from build123d import *

# Parameters (mm, degrees)
SKETCH1_R          = 6.35
BASE_EXTRUDE_DEPTH = 1.5875
CHAMFER1_SIZE      = 0.254


with BuildPart() as part:
    # Sketch1 → Base-Extrude (new body, symmetric)
    with BuildSketch(Plane(origin=(0, 0, 0), x_dir=(1, 0, 0), z_dir=(0, 1, 0))):
        with BuildLine():
            Line((6.35, 0), (6.35, 104.775))
            ThreePointArc((6.35, 104.775), (12.7, 111.125), (19.05, 104.775))
            Line((19.05, 104.775), (19.05, -31.75))
            ThreePointArc((19.05, -31.75), (0, -50.8), (-19.05, -31.75))
            Line((-19.05, -31.75), (-19.05, 104.775))
            ThreePointArc((-19.05, 104.775), (-12.7, 111.125), (-6.35, 104.775))
            Line((-6.35, 104.775), (-6.35, 0))
            ThreePointArc((-6.35, 0), (0, -6.35), (6.35, 0))
        make_face()
        with Locations(Location((0, -31.75, 0), (0, 0, 270))):  # turned: the seam where the file's is
            Circle(SKETCH1_R, mode=Mode.SUBTRACT)
    extrude(amount=BASE_EXTRUDE_DEPTH, both=True)

    # Chamfer1
    chamfer1_edges = [part.edges().sort_by_distance(p)[0] for p in [
        (-12.7, 1.5875, -111.125),
        (-6.35, -1.5875, -52.3875),
        (0, -1.5875, 6.35),
        (-19.05, 1.5875, -36.5125),
        (0, 1.5875, 50.8),
        (19.05, 1.5875, -36.5125),
        (0, -1.5875, 25.4),
        (0, 1.5875, 25.4),
        (12.7, 1.5875, -111.125),
        (6.35, 1.5875, -52.3875),
        (0, 1.5875, 6.35),
        (-6.35, 1.5875, -52.3875),
        (6.35, -1.5875, -52.3875),
        (12.7, -1.5875, -111.125),
        (19.05, -1.5875, -36.5125),
        (0, -1.5875, 50.8),
        (-19.05, -1.5875, -36.5125),
        (-12.7, -1.5875, -111.125),
    ]]
    chamfer(chamfer1_edges, length=CHAMFER1_SIZE)


solid = part.part
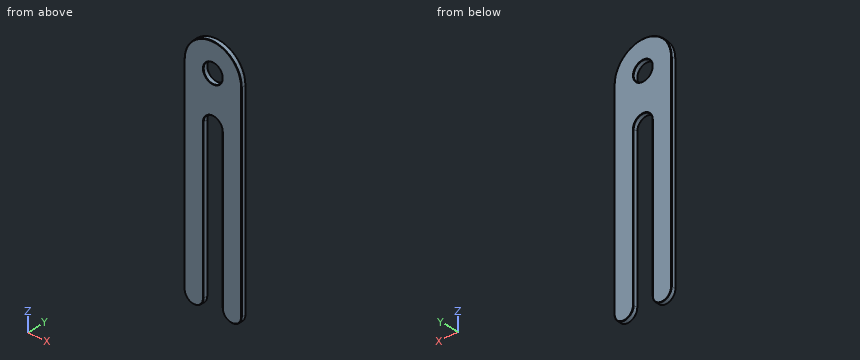
Input: part model. Units: mm. Frame: model coordinates. Give positions to 0.01 mm unless a question says otherwise; leave off trailing zeros. Order: outer loops, then holes, each group sorted by start corner. A loop starts at its lowest first (then second) coordinate and runs counter-clockwise, first axis right, second up. Notation, with made-up numbers: (42, 61.5) - (57, 61.5) arc R16 cw to (57, 75.5) - close; hole circle Ø11 at (55.5, -6.75). An arc over 180 degrees is marked (long way). Answer as a JSON object with one key per item and string values. Group by question number.
Q1. Line query: probe 1 along X at (y, z) = (-0.1, -49); probe 2 along Z at (x, y) = (-1.5, -0.5). Output: solid intervals per line, ascending.
Q2. Cut plane B-B, the plane z = -87.5. Output: boundary loops of the cut face in (x, y), then the cut area to 3 significant figures.
Q3. Cut plane A-A, the plane x = 0. Output: boundary loops of the cut face in (y, z).
Q4. Cut plane C-C, the plane y = 0.35. Output: boundary loops of the cut face in (x, z) (3 decimals).
Results:
{
 "1": {"probe 1": "-19.05 to -6.35, 6.35 to 19.05", "probe 2": "6.17 to 25.58, 37.92 to 50.74"},
 "2": {"outline": "(-19.05, -1.33) - (-18.8, -1.59) - (-6.6, -1.59) - (-6.35, -1.33) - (-6.35, 1.33) - (-6.6, 1.59) - (-18.8, 1.59) - (-19.05, 1.33) - close; (6.35, -1.33) - (6.6, -1.59) - (18.8, -1.59) - (19.05, -1.33) - (19.05, 1.33) - (18.8, 1.59) - (6.6, 1.59) - (6.35, 1.33) - close", "area": "80.4 mm^2"},
 "3": {"outline": "(-1.59, 6.6) - (-1.33, 6.35) - (1.33, 6.35) - (1.59, 6.6) - (1.59, 25.15) - (1.33, 25.4) - (-1.33, 25.4) - (-1.59, 25.15) - close; (-1.59, 38.35) - (-1.33, 38.1) - (1.33, 38.1) - (1.59, 38.35) - (1.59, 50.55) - (1.33, 50.8) - (-1.33, 50.8) - (-1.59, 50.55) - close"},
 "4": {"outline": "(-19.05, -104.775) arc R6.35 ccw to (-6.35, -104.775) - (-6.35, 0) arc R6.35 cw to (6.35, 0) - (6.35, -104.775) arc R6.35 ccw to (19.05, -104.775) - (19.05, 31.75) arc R19.05 ccw to (-19.05, 31.75) - close; hole circle Ø12.7 at (0, 31.75)"}
}
